CAD build for the part. Positions are in the model's coordinates, mm. A direction names the side the tool comes from. Give positions to 0.01 mm unless a question says otherwise; leave off trailing zeros. Loops run counter-clockwise (first coordinate to the right, second up) from the corner with the lowest first, then second, coordinate; pieces in that order, holes last. Notation, with made-up numbers: M 48,19 L 65,19 A27 cw 65,58 Z; hole C 28.25,-39 d10. An arc over 180 degrees is marked long. Answer as CSV lines item,"result".
Autodesk Inventor part; units mm, degrees
ref_plane "YZ Plane" through (0, 0, 0) normal (1, 0, 0) x (0, 1, 0)
ref_plane "XZ Plane" through (0, 0, 0) normal (0, 1, 0) x (-1, 0, 0)
ref_plane "XY Plane" through (0, 0, 0) normal (0, 0, 1) x (1, 0, 0)
sketch "Sketch1" plane through (0, 0, 0) normal (0, 1, 0) x (-1, 0, 0)
  circle A0 centre (0, 0) radius 38.1
  line L0 (-20.32, 68.58) -> (350.52, 68.58)
  line L1 (381, 38.1) -> (381, -38.1)
  line L2 (350.52, -68.58) -> (-20.32, -68.58)
  line L3 (-50.8, -38.1) -> (-50.8, 38.1)
  arc A1 (-20.32, 68.58) -> (-50.8, 38.1) centre (-20.32, 38.1) ccw
  arc A2 (-50.8, -38.1) -> (-20.32, -68.58) centre (-20.32, -38.1) ccw
  arc A3 (381, 38.1) -> (350.52, 68.58) centre (350.52, 38.1) ccw
  arc A4 (350.52, -68.58) -> (381, -38.1) centre (350.52, -38.1) ccw
  point P0 (-50.8, 68.58)
  point P1 (381, -68.58)
  point P2 (-50.8, -68.58)
  dimension "d0" = 76.2
  dimension "d1" = 137.16
  dimension "d2" = 431.8
  dimension "d3" = 50.8
  dimension "d4" = 68.58
  dimension "d5" = 30.48
extrude "Extrusion1" add sketch "Sketch1" against normal blind 129.54
sketch "Sketch2" plane through (0, -129.54, 0) normal (0, -1, 0) x (1, 0, 0)
  circle A0 centre (0, 0) radius 38.1
  dimension "d17" = 76.2
extrude "Extrusion2" add sketch "Sketch2" against normal blind 93.98
sketch "Sketch3" plane through (0, 0, 0) normal (0, 1, 0) x (1, 0, 0)
  line L0 (50.8, 38.1) -> (50.8, -38.1)
  line L1 (50.8, 0) -> (-132.08, 0)
  line L2 (20.32, -68.58) -> (-350.52, -68.58)
  line L3 (-132.08, -68.58) -> (-434.975, -68.58)
  line L4 (-434.975, -68.58) -> (-434.975, 68.58)
  line L5 (-434.975, 68.58) -> (-132.08, 68.58)
  line L6 (-132.08, 68.58) -> (-132.08, -68.58)
  point P0 (0, 0)
  dimension "d10" = 182.88
extrude "Extrusion3" cut sketch "Sketch3" against normal blind 35.2425
sketch "Sketch4" plane through (0, -35.2425, 0) normal (0, 1, 0) x (1, 0, 0)
  line L0 (-381, -38.1) -> (-381, 38.1)
  line L1 (-381, 0) -> (-328.6125, 0)
  line L2 (-381, 0) -> (-317.5, 0)
  circle A0 centre (-317.5, 0) radius 30.48
  point P0 (0, 0)
  dimension "d14" = 60.96
  dimension "d18" = 317.5
extrude "Extrusion4" add sketch "Sketch4" along normal blind 63.5
properties part number "Shoulder2 Link-lrg"
Q1. Pin check, flat tips, straight feed: P1, Ø2, axis at x = -216.5, z = 17, coming from the +Y side; P2, Ø8, axis at y = -69, z = -52.5, coming from the -X side; P3, Ø6, axis at y = -17, z = 22.5, coming from the -X side. Stop position of each tip, or through.
Solution:
P1,"stops at y = -35.24"
P2,"stops at x = -379.17"
P3,"stops at x = -340.93"
Q2. Wall check: line 1 (Z direction, x = 0, y = -17); line 2 (Y direction, x = -347, z = 58.5); line 3 (X direction, y = -31, z = -11). Give the ranges that are in metal, low to high. Write a range as [from, to].
Solution:
line 1,"z = [-68.58, -38.1], [38.1, 68.58]"
line 2,"y = [-129.54, -35.24]"
line 3,"x = [-345.93, -289.07], [-132.08, -36.48], [36.48, 50.8]"
Q3. Mould opens along X. For faces 4 (the flat face through (-132.08, -17, -1)), 5 (the flat face through (-381, -82, 1)), 6 (the cylindrical face through (41.63, -63.86, 59.89)) say: released by +X, released by -X, zero draft, split by the parting line, or undercut.
Solution:
face 4,"undercut"
face 5,"released by -X"
face 6,"released by +X"
Q4. Cut at A-A (y = -7.5). Write the cut outline in (x, z), and give its area (3 significant figures).
Solution:
outline,"C -317.5,0 d60.96; M -132.08,-68.58 L 20.32,-68.58 A30.48 ccw 50.8,-38.1 L 50.8,38.1 A30.48 ccw 20.32,68.58 L -132.08,68.58 Z; hole C 0,0 d76.2"
area,"23,000 mm²"
Q5. Cut at D-D (x = -171.5). Write the cut outline in (y, z).
Solution:
outline,"M -129.54,-68.58 L -35.24,-68.58 L -35.24,68.58 L -129.54,68.58 Z"
Q6. Which spindle directions (+Z, -Z, +X, -X, +Y, -Y) get a long thin tool onto all of the face, cutting with end or side? Do faces 1 (the flat face through (-60, 0, 1)), 2 (the cylindrical face through (-372.31, -81.73, 59.41)), 3 (the cylindrical face through (30.235, -17.531, -23.183)). Say none if no direction does.
Solution:
face 1,"+Z, -Z, +X, +Y"
face 2,"+Z, -X, +Y, -Y"
face 3,"+Y"
Q7. Cut at C-C (z = 13). Write the cut outline in (x, y), and give its area (3 significant figures).
Solution:
outline,"M -381,-129.54 L 50.8,-129.54 L 50.8,0 L 35.81,0 L 35.81,-35.56 L -35.81,-35.56 L -35.81,0 L -132.08,0 L -132.08,-35.24 L -289.93,-35.24 L -289.93,28.26 L -345.07,28.26 L -345.07,-35.24 L -381,-35.24 Z"
area,"48,100 mm²"
Q8. Cut at B-B (x = 0). Write the cut outline in (y, z), and give its area (3 significant figures).
Solution:
outline,"M -129.54,-68.58 L 0,-68.58 L 0,-38.1 L -35.56,-38.1 L -35.56,38.1 L 0,38.1 L 0,68.58 L -129.54,68.58 Z"
area,"15,100 mm²"
